from build123d import *

# Parameters (mm, degrees)
SKETCH1_R           = 1.7
SKETCH1_R_2         = 2
BOSS_EXTRUDE1_DEPTH = 6


with BuildPart() as part:
    # Sketch1 → Boss-Extrude1 (new body)
    with BuildSketch(Plane.XY):
        with BuildLine():
            Line((-12, 23), (-6, 23))
            ThreePointArc((-6, 23), (-3.878679656, 22.121320344), (-3, 20))
            Line((-3, 20), (-3, 18))
            ThreePointArc((-3, 18), (0, 15), (3, 18))
            Line((3, 18), (3, 20))
            ThreePointArc((3, 20), (3.878679656, 22.121320344), (6, 23))
            Line((6, 23), (12, 23))
            ThreePointArc((12, 23), (14.121320344, 22.121320344), (15, 20))
            Line((15, 20), (15, -20))
            ThreePointArc((15, -20), (14.121320344, -22.121320344), (12, -23))
            Line((12, -23), (6, -23))
            ThreePointArc((6, -23), (3.878679656, -22.121320344), (3, -20))
            Line((3, -20), (3, -18))
            ThreePointArc((3, -18), (0, -15), (-3, -18))
            Line((-3, -18), (-3, -20))
            ThreePointArc((-3, -20), (-3.878679656, -22.121320344), (-6, -23))
            Line((-6, -23), (-12, -23))
            ThreePointArc((-12, -23), (-14.121320344, -22.121320344), (-15, -20))
            Line((-15, -20), (-15, 20))
            ThreePointArc((-15, 20), (-14.121320344, 22.121320344), (-12, 23))
        make_face()
        with Locations((-9, 18.5)):
            Circle(SKETCH1_R, mode=Mode.SUBTRACT)
        with Locations(Location((9, 18.5, 0), (0, 0, 180))):
            Circle(SKETCH1_R, mode=Mode.SUBTRACT)
        with Locations((9, -18.5)):
            Circle(SKETCH1_R, mode=Mode.SUBTRACT)
        with Locations(Location((-9, -18.5, 0), (0, 0, 180))):
            Circle(SKETCH1_R, mode=Mode.SUBTRACT)
        with Locations((-5, 10.5)):
            Circle(SKETCH1_R_2, mode=Mode.SUBTRACT)
        with Locations(Location((5, 10.5, 0), (0, 0, 180))):
            Circle(SKETCH1_R_2, mode=Mode.SUBTRACT)
        with Locations((5, -10.5)):
            Circle(SKETCH1_R_2, mode=Mode.SUBTRACT)
        with Locations(Location((-5, -10.5, 0), (0, 0, 180))):
            Circle(SKETCH1_R_2, mode=Mode.SUBTRACT)
    extrude(amount=BOSS_EXTRUDE1_DEPTH)


solid = part.part
Build history of the part. All positions in model axes, mm. A direction names the side the tool comes from. Coordinates: 2 decimals unless noted, no trailing zeros. Order: outer loops, then holes, each group sorted by start corner. A loop starts at its lowest first (then second) coordinate and runs counter-clockwise, first axis right, second up. Notation, with made-up numbers: M 63,84.25 L 103,84.25 A27 ccw 103,116.25 Z; hole C 34.25,-35.75 d3. An arc over 180 degrees is marked long. One line per question, with ' | ' between items. Start each with the question number.
Q1. Saw through at D-D (y = -10.5). List the corners of the cut face in (x, z), then the cut area to 3 significant figures.
Q2. Two-plate mould, pull along Y, no slides. Class faces 1 (the face through (3, -19, 3)), 2 (the face through (-3.86, -22.1, 2.96)), 3 (the face through (-3.526, -11.852, 2.958)), 4 (the face through (-8.779, -20.186, 2.958)): +Y half, -Y half, draft (parallel to the pull), parting line (faces both ways), or undercut.
Q3. Saw through at B-B (y = -18.5). List the corners of the cut face in (x, z).
Q4. 3-axis set-ups, long thin cutter, end or side, ignore diameter. For faces 5 (the face through (3, 19, 3)), 6 (the face through (3.9, -22.14, 2.96)), 7 (the face through (6.474, 9.148, 2.958)): which of +Z, -Z, +X, -X, +Y, -Y reach the whole face in a straight line?
Q5. Saw through at C-C (z = 4.9). Count the separate pieces of the cut face and the enclosed holes in it, then the cut area to 3 significant figures.
Q6. Probe L1, parallel to Y at x = -9, z = 4.75; L2, parallel to Y at x = 10.5, z = 5.55; L3, parallel to X at y = -17.5, z = 1.55. List the from-to ranges inside material, lowest first. Write a range as from..to.
Q7. Saw through at A-A (x = -9). List the corners of the cut face in (y, z), then the cut area to 3 significant figures.
Check values:
1) outline: M -15,0 L -7,0 L -7,6 L -15,6 Z; M -3,0 L 3,0 L 3,6 L -3,6 Z; M 7,0 L 15,0 L 15,6 L 7,6 Z | area: 132 mm2
2) face 1: draft | face 2: -Y half | face 3: undercut | face 4: undercut
3) outline: M -15,0 L -10.7,0 L -10.7,6 L -15,6 Z; M -7.3,0 L -3,0 L -3,6 L -7.3,6 Z; M 3,0 L 7.3,0 L 7.3,6 L 3,6 Z; M 10.7,0 L 15,0 L 15,6 L 10.7,6 Z
4) face 5: +Z, -Z, +Y | face 6: +Z, -Z, -Y | face 7: +Z, -Z
5) separate pieces: 1 | enclosed holes: 8 | area: 1,190 mm2
6) L1: y = -23..-20.2, -16.8..16.8, 20.2..23 | L2: y = -23..-19.3, -17.7..17.7, 19.3..23 | L3: x = -15..-10.37, -7.63..-2.96, 2.96..7.63, 10.37..15
7) outline: M -23,0 L -20.2,0 L -20.2,6 L -23,6 Z; M -16.8,0 L 16.8,0 L 16.8,6 L -16.8,6 Z; M 20.2,0 L 23,0 L 23,6 L 20.2,6 Z | area: 235 mm2
